from build123d import *

# Parameters (mm, degrees)
F0_W     = 25.4
F0_H     = 19.05
F1_DEPTH = 25.4
F3_DEPTH = 14.2875
F5_D     = 2.7051
F7_D     = 11.90498
F8_R     = 3.175
F9_R     = 0.762


with BuildPart() as f1:
    # F0 (on Top) → F1 (new body)
    with BuildSketch(Plane.XY):
        Rectangle(F0_W, F0_H)
    extrude(amount=F1_DEPTH)

    # F2 (on face) → F3 (cut)
    with BuildSketch(Plane.XZ.offset(9.525)):
        with BuildLine():
            Line((6.731, 25.4), (-6.731, 25.4))
            Line((-6.731, 25.4), (-6.731, 18.796))
            ThreePointArc((-6.731, 18.796), (0, 12.065), (6.731, 18.796))
            Line((6.731, 18.796), (6.731, 25.4))
        make_face()
    extrude(amount=-F3_DEPTH, mode=Mode.SUBTRACT)

    # F5 (through all)
    with Locations(Plane.XY.offset(25.4)):
        with Locations((-8.73125, 4.7625), (-8.73125, -4.7625), (8.73125, 4.7625), (8.73125, -4.7625)):
            Hole(F5_D / 2)

    # F7 (through all)
    with Locations(Plane.XZ.offset(-4.7625)):
        with Locations((0, 18.796)):
            Hole(F7_D / 2)

    # F8
    f8_edges = [f1.edges().sort_by_distance(p)[0] for p in [
        (-12.7, -9.525, 12.7),
        (12.7, -9.525, 12.7),
        (12.7, 9.525, 12.7),
        (-12.7, 9.525, 12.7),
    ]]
    fillet(f8_edges, radius=F8_R)

    # F9
    f9_edges = [f1.edges().sort_by_distance(p)[0] for p in [
        (-6.731, 4.7625, 22.098),
        (0, 4.7625, 12.065),
        (6.731, 4.7625, 22.098),
    ]]
    fillet(f9_edges, radius=F9_R)


solid = f1.part
Can you work these out from the model? Positions are in its coordinate system, mm. A direction names the side the tool comes from. Round coordinates to 2 decimals unless told otherwise and drop trailing zeros. Write each loop counter-clockwise with the first axis right and the second up, starting at its lowest first coordinate (ties: lowest second). Pieces come first, ordered by that corner, then holes. Notation, with made-up numbers: M 62,-20.5 L 74,-20.5 A28 cw 74,9.5 Z; hole C 84.25,-32 d4. An arc over 180 degrees is marked long. Use CSV: the item, a comma, the result in double quotes.
(1) Imagine slicing it at D-D (z = 3.75). Count the separate pieces of the cut face and the enclosed holes in it, plus the area to 3 significant figures.
Check values:
separate pieces,"1"
enclosed holes,"4"
area,"452 mm^2"
(2) Imagine slicing it at B-B (y = -3.75). Write out the boundary of the cut face in (x, z), plus the area to 3 significant figures.
Check values:
outline,"M -12.7,0 L -9.63,0 L -9.63,25.4 L -12.7,25.4 Z; M -7.83,0 L 7.83,0 L 7.83,25.4 L 6.73,25.4 L 6.73,18.8 A6.73 cw -6.73,18.8 L -6.73,25.4 L -7.83,25.4 Z; M 9.63,0 L 12.7,0 L 12.7,25.4 L 9.63,25.4 Z"
area,"394 mm^2"
(3) We'd pull the mould along Y, two halves only. Please class faces 1 (the flat face through (0, 4.762, 25)), 2 (the cylindrical face through (10.082, 4.822, 12.522)), 3 (the flat face through (0, 0, 0)), 4 (the cylindrical face through (9.73, -3.85, 12.52)): +Y half, -Y half, draft (parallel to the pull), parting line (faces both ways), or undercut.
Check values:
face 1,"-Y half"
face 2,"undercut"
face 3,"draft"
face 4,"undercut"
(4) I need wall thicknesses on line 1 along Y through (x, z) = (-9, 12) (3 decimals); line 2 along X through (y, z) = (1.25, 21.5); line 3 along Y through (x, z) = (7.5, 19) (3 decimals). Which ranges of each line are inside material? Lowest first, please.
Check values:
line 1,"-9.525 to -6.088, -3.437 to 3.437, 6.088 to 9.525"
line 2,"-12.7 to -6.73, 6.73 to 12.7"
line 3,"-9.525 to -5.322, -4.203 to 4.203, 5.322 to 9.525"
(5) On a 3-axis mill with a long thin cutter (end or side, diameter ignored), from which of +Z, -Z, +X, -X, +Y, -Y can I reach the whole of each face in a straight line? I mean faces 5 (the cylindrical face through (-0.148, -2.857, 12.067)), 6 (the flat face through (0, -9.525, 10)). Say none if no direction works.
Check values:
face 5,"+Z, -Y"
face 6,"+Z, -Z, +X, -X, -Y"
(6) Imagine slicing it at C-C (x = -9). Write out the boundary of the cut face in (y, z) (3 decimals), plus the area to 3 significant figures.
Check values:
outline,"M -9.525,0 L -6.088,0 L -6.088,25.4 L -9.525,25.4 Z; M -3.437,0 L 3.437,0 L 3.437,25.4 L -3.437,25.4 Z; M 6.088,0 L 9.525,0 L 9.525,25.4 L 6.088,25.4 Z"
area,"349 mm^2"
(7) I'm going to push flat-ended pins straight in: pin 1 (13 mm diameter, centred on x = -2.5, z = 18.5, fed in from -Y) (3 decimals); pin 2 (3 mm diameter, centred on x = 3.5, y = -3.5, fed in from +Z). Where does each tip first touch, or does it pass through?
Check values:
pin 1,"y = -9.525"
pin 2,"z = 14.29"
